from build123d import *

# Parameters (mm, degrees)
F0_R     = 70
F1_DEPTH = 70
F3_R     = 25
F4_DEPTH = 25
F5_R     = 62.5
F6_DEPTH = 3


with BuildPart() as f1:
    # F0 (on Top) → F1 (new body)
    with BuildSketch(Plane.XY):
        with Locations((-43.56515, 8.154014)):
            Circle(F0_R)
    extrude(amount=F1_DEPTH)

    # F3 (on offset) → F4 (cut)
    with BuildSketch(Plane.XZ.offset(62)):
        with Locations((-50.681688, 37.782334)):
            Circle(F3_R)
    extrude(amount=-F4_DEPTH, mode=Mode.SUBTRACT)

    # F5 (on face) → F6 (cut)
    with BuildSketch(Plane.XY.offset(70)):
        with Locations((-43.56515, 8.154014)):
            Circle(F5_R)
    extrude(amount=-F6_DEPTH, mode=Mode.SUBTRACT)


solid = f1.part
CAD build for the part. Positions are in the model's coordinates, mm. A direction names the side the tool comes from. Round coordinates to 2 decimals unless told otherwise and drop trailing zeros. Order: outer loops, then holes, each group sorted by start corner. A loop starts at its lowest first (then second) coordinate and runs counter-clockwise, first axis right, second up. Notation, with made-up numbers: (-29.75, 40) - (15.25, 40) arc R24 cw to (15.25, 64) - close; hole circle Ø11 at (82.5, -33). An arc over 180 degrees is marked (long way). Return JSON: item names as keys, results as strings.
(1) Pin check, flat tips, straight feed: pin 1 Ø4 at (y, z) = (3.5, 62.5) entering from -X; pin 2 Ø1.5 at (x, z) = (-16.5, 26.5) entering from -Y; pin 3 Ø4 at (x, z) = (-60, 18) entering from -Y. Stop position of each tip, or through.
Answer key:
{"pin 1": "stops at x = -113.51", "pin 2": "stops at y = -56.71", "pin 3": "stops at y = -37"}
(2) Cut at A-A (x = -14.5). Give the cut face in (y, z).
Answer key:
{"outline": "(-55.53, 0) - (71.83, 0) - (71.83, 70) - (63.48, 70) - (63.48, 67) - (-47.18, 67) - (-47.18, 70) - (-55.53, 70) - close"}
(3) Pull direction Z, two halves, no side cores. Call faces 4 (the face through (-70, 66, 70)), 5 (the face through (-27.588, -49.598, 28.207)), 6 (the face through (14.17, -15.78, 68.52)): +Z half, -Z half, draft (parallel to the pull), parting line (faces both ways), or undercut.
Answer key:
{"face 4": "+Z half", "face 5": "undercut", "face 6": "draft"}
(4) Cut at D-D (z = 52.5). Give the cut face in (x, y), then the cut area to 3 significant figures.
Answer key:
{"outline": "(-70.89, -56.29) - (-70.89, -37) - (-30.47, -37) - (-30.47, -60.61) arc R70 ccw (long way) to start", "area": "14,400 mm^2"}
(5) Cut at B-B (y = -43). Give the cut face in (x, z) (3 decimals).
Answer key:
{"outline": "(-91.349, 0) - (4.218, 0) - (4.218, 70) - (-7.655, 70) - (-7.655, 67) - (-79.475, 67) - (-79.475, 70) - (-91.349, 70) - close; hole circle Ø50 at (-50.682, 37.782)"}
(6) Tool access for faces 1 (the face through (-44, 9, 67)), 2 (the face through (-52.68, 77.56, 34.51)), 3 (the face through (-51, -37, 38)): list every direction of +Z, -Z, +X, -X, +Y, -Y with a clear straight run to the whole face (end or side of a thin tool).
Answer key:
{"face 1": "+Z", "face 2": "+Z, -Z", "face 3": "-Y"}
(7) Wall check: probe 1 along Z at (x, y) = (-13, 60); probe 2 along Z at (x, y) = (-47, -44); probe 3 along X at (y, z) = (-52.5, 39.5). Give the ranges that are in metal, low to high. Write a range as from..to.
Answer key:
{"probe 1": "z = 0..67", "probe 2": "z = 0..13.05, 62.51..67", "probe 3": "x = -78.51..-75.62, -25.74..-8.62"}
(8) Cut at C-C (y = 44.5). Give the cut face in (x, z), then the cut area to 3 significant figures.
Answer key:
{"outline": "(-103.39, 0) - (16.26, 0) - (16.26, 70) - (7.28, 70) - (7.28, 67) - (-94.41, 67) - (-94.41, 70) - (-103.39, 70) - close", "area": "8,070 mm^2"}
